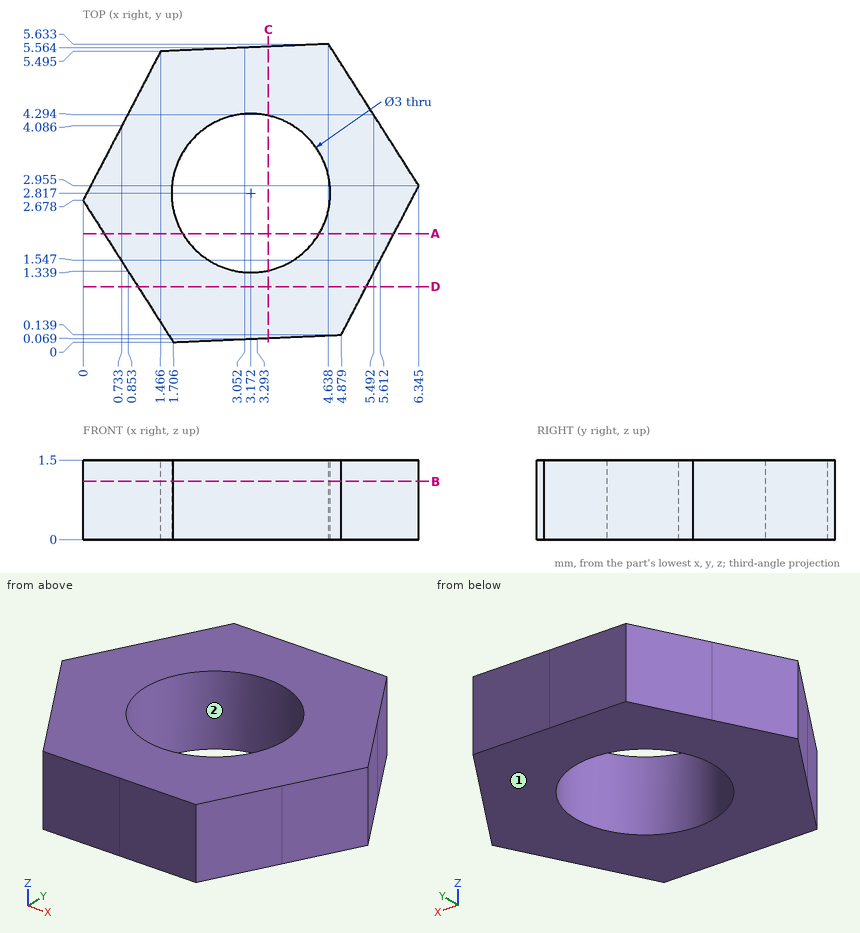
Verification items for this drawing (mm, ordinates from the low corner). Give positions to 0.01 mm unless a question says otherwise; leave off trailing zeros. Loops run counter-clockwise (first coordinate to the right, second up) from the corner with the lowest first, then second, coordinate; pieces in that order, holes last. Notation, with made-up numbers: M 58.25,11 L 85.25,11 A26 ccw 85.25,28 Z; hole C 80.25,40 d5. An arc over 180 degrees is marked long. Answer in a Markdown table with one row per item.
1) Cross-section at C-C (x = 3.5). Enter the section's corners in (y, z).
Solutions:
| item | result |
|---|---|
| outline | M 0.08,0 L 1.35,0 L 1.35,1.5 L 0.08,1.5 Z; M 4.28,0 L 5.58,0 L 5.58,1.5 L 4.28,1.5 Z |
2) Thickness scan on line 1 (Y direction, x = 3.25, z = 1.1) (1 decimal); line 2 (X direction, y = 1.55, z = 1.45) (1 decimal); line 3 (Y direction, x = 2.25, z = 1.2) (1 decimal). Record the ranges inside material, lowest first.
Solutions:
| item | result |
|---|---|
| line 1 | y = 0.1 to 1.3, 4.3 to 5.6 |
| line 2 | x = 0.7 to 2.4, 4 to 5.6 |
| line 3 | y = 0 to 1.6, 4 to 5.5 |
3) Cross-section at D-D (y = 1.05). Enter the section's corners in (x, z).
Solutions:
| item | result |
|---|---|
| outline | M 1.04,0 L 5.35,0 L 5.35,1.5 L 1.04,1.5 Z |
4) Cross-section at A-A (y = 2.05). Enter the section's corners in (x, z).
Solutions:
| item | result |
|---|---|
| outline | M 0.4,0 L 1.88,0 L 1.88,1.5 L 0.4,1.5 Z; M 4.46,0 L 5.87,0 L 5.87,1.5 L 4.46,1.5 Z |
5) Mould release check, pull along Y, two halves, no side actions. Record for the marked faces 1 and 2: released by +Y, released by -Y, zero draft, split by the parting line, or undercut.
Solutions:
| item | result |
|---|---|
| face 1 | zero draft |
| face 2 | undercut |
6) Cross-section at B-B (z = 1.1). Enter the section's corners in (x, y) (1 decimal).
Solutions:
| item | result |
|---|---|
| outline | M 0,2.7 L 1.7,0 L 4.9,0.1 L 6.3,3 L 4.6,5.6 L 1.5,5.5 Z; hole C 3.2,2.8 d3 |
